```python
from build123d import *

# Parameters (mm, degrees)
SKETCH_1_R          = 1.5
EXTRUDE_1_DEPTH     = 8
SKETCH_2_R          = 1.5
CUT_EXTRUDE_1_DEPTH = 28.367864367
SKETCH_3_R          = 3
CUT_EXTRUDE_2_DEPTH = 3
CUT_EXTRUDE_3_DEPTH = 3


with BuildPart() as part:
    # 草图1 → 凸台-拉伸1 (new body)
    with BuildSketch(Plane(origin=(0, 0, 0), x_dir=(1, 0, 0), z_dir=(0, 1, 0))):
        Polygon((-18, 19), (18, 19), (18, 6), (10, 6), (10, 0), (-10, 0), (-10, 6), (-18, 6), align=None)
        with Locations(Location((7.5, 14.5, 0), (0, 0, 270))):
            Circle(SKETCH_1_R, mode=Mode.SUBTRACT)
        with Locations(Location((7.5, 4.5, 0), (0, 0, 90))):
            Circle(SKETCH_1_R, mode=Mode.SUBTRACT)
        with Locations(Location((-7.5, 4.5, 0), (0, 0, 270))):
            Circle(SKETCH_1_R, mode=Mode.SUBTRACT)
        with Locations(Location((-7.5, 14.5, 0), (0, 0, 90))):
            Circle(SKETCH_1_R, mode=Mode.SUBTRACT)
    extrude(amount=EXTRUDE_1_DEPTH)

    # 草图2 → 切除-拉伸1 (cut, through all)
    with BuildSketch(Plane(origin=(0, 0, -19), x_dir=(-1, 0, 0), z_dir=(0, 0, -1))):
        with Locations((-14, 4)):
            Circle(SKETCH_2_R)
        with Locations((14, 4)):
            Circle(SKETCH_2_R)
    extrude(amount=-CUT_EXTRUDE_1_DEPTH, mode=Mode.SUBTRACT)

    # 草图3 → 切除-拉伸2 (cut)
    with BuildSketch(Plane.XZ):
        with Locations(Location((-7.5, -14.5, 0), (0, 0, 270))):
            Circle(SKETCH_3_R)
        with Locations(Location((7.5, -14.5, 0), (0, 0, 270))):
            Circle(SKETCH_3_R)
    extrude(amount=-CUT_EXTRUDE_2_DEPTH, mode=Mode.SUBTRACT)

    # 草图4 → 切除-拉伸3 (cut)
    with BuildSketch(Plane.XZ):
        with BuildLine():
            ThreePointArc((-10, -2.841687605), (-6.633974596, -1.627718677), (-4.5, -4.5))
            Line((-4.5, -4.5), (-4.5, 0))
            Line((-4.5, 0), (-10, 0))
            Line((-10, 0), (-10, -2.841687605))
        make_face()
        with BuildLine():
            Line((-6, -4.5), (-4.5, -4.5))
            ThreePointArc((-4.5, -4.5), (-6.633974596, -1.627718677), (-10, -2.841687605))
            Line((-10, -2.841687605), (-10, -4.5))
            Line((-10, -4.5), (-9, -4.5))
            ThreePointArc((-9, -4.5), (-7.5, -3), (-6, -4.5))
        make_face()
        with BuildLine():
            ThreePointArc((-10.098076211, -6), (-6.723542865, -7.397777479), (-4.5, -4.5))
            Line((-4.5, -4.5), (-6, -4.5))
            ThreePointArc((-6, -4.5), (-7.5, -6), (-9, -4.5))
            Line((-9, -4.5), (-10, -4.5))
            Line((-10, -4.5), (-10, -6))
            Line((-10, -6), (-10.098076211, -6))
        make_face()
        with BuildLine():
            ThreePointArc((10, -2.841687605), (6.633974596, -1.627718677), (4.5, -4.5))
            Line((4.5, -4.5), (6, -4.5))
            ThreePointArc((6, -4.5), (7.5, -3), (9, -4.5))
            Line((9, -4.5), (10, -4.5))
            Line((10, -4.5), (10, -2.841687605))
        make_face()
        with BuildLine():
            Line((6, -4.5), (4.5, -4.5))
            ThreePointArc((4.5, -4.5), (6.723542865, -7.397777479), (10.098076211, -6))
            Line((10.098076211, -6), (10, -6))
            Line((10, -6), (10, -4.5))
            Line((10, -4.5), (9, -4.5))
            ThreePointArc((9, -4.5), (7.5, -6), (6, -4.5))
        make_face()
        with BuildLine():
            Line((10, 0), (4.5, 0))
            Line((4.5, 0), (4.5, -4.5))
            ThreePointArc((4.5, -4.5), (6.633974596, -1.627718677), (10, -2.841687605))
            Line((10, -2.841687605), (10, 0))
        make_face()
    extrude(amount=-CUT_EXTRUDE_3_DEPTH, mode=Mode.SUBTRACT)


solid = part.part
```
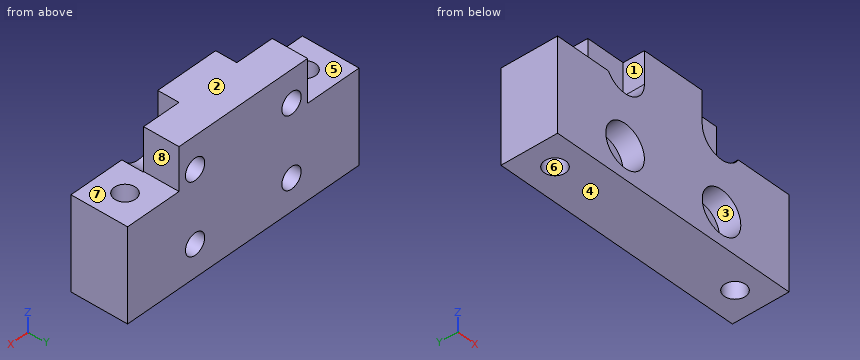
Geometry: final body of the model. Coordinates: model frame, mm. Face numbers are marked on the shaded views. A direction names the side the tool comes from. Round coordinates to 2 decimals unless told otherwise and drop trailing zeros. Write each loop counter-clockwise with the first axis right and the second up, starting at its lowest first coordinate (ties: lowest second). Pieces come first, ordered by that corner, then holes.
Item 1: Mould query, pull axis X, two halves, no side actions, for the marked faces 6, 7 and 8. Classes: +X half, -X half, draft (parallel to the pull), parting line (faces both ways), or undercut.
Item 2: Set-up query: the marked faces 1, 2, 3, 4 and 5. Return all of +Z, -Z, +X, -X, +Y, -Y with unobstructed straight access to the full face (end or side cutting, diameter ignored); none if empty.
Item 3: Material intervals for L1, parallel to Z at x = 7.5, y = 4.5; L2, parallel to X at y = 6.65, z = -4.5; L3, parallel to X at y = 0.8, z = -14.5, sorted ascending.
Item 4: Section query D-D (x = 7.5). Return loops of the section in (y, z).
Item 5: Section query B-B (x = 14). Return loops of the section in (y, z).
Item 6: Section query A-A (y = 4). Return loops of the section in (x, z), plus the area to 3 significant figures.
Item 7: Section query C-C (z = -14.5). Return loops of the section in (x, y), plus the area to 3 significant figures.
Item 8: Pin query (flat end, axial travel): P1, Ø4, axis at x = 3, y = 4, coming from the +Z side; P2, Ø5, axis at x = -7.5, z = -14.5, coming from the -Y side; P3, Ø2.5, axis at x = -7.5, z = -14.5, coming from the +Y side; P4, Ø0.9, axis at y = 2, z = -1.5, coming from the -X side. Return the tip coordinate at first contact, or that it passes through.
Completed:
1. face 6: undercut
1. face 7: draft
1. face 8: +X half
2. face 1: +Z, -X, -Y
2. face 2: +Z, +X, -X, +Y, -Y
2. face 3: -Y
2. face 4: -Z, +X, -X, +Y, -Y
2. face 5: +Z, -X, +Y, -Y
3. L1: z = -19 to -16, -13 to -6, -3 to 0
3. L2: x = -10 to -9, -6 to 6, 9 to 10
3. L3: x = -18 to -10.5, -4.5 to 4.5, 10.5 to 18
4. outline: (0, -19) - (8, -19) - (8, -16) - (3, -16) - (3, -17.5) - (0, -17.5) - close; (0, -11.5) - (3, -11.5) - (3, -13) - (8, -13) - (8, -6) - (3, -6) - (3, -7.5) - (0, -7.5) - close; (3, -3) - (8, -3) - (8, 0) - (3, 0) - close
5. outline: (0, -19) - (2.5, -19) - (2.5, -6) - (0, -6) - close; (5.5, -19) - (8, -19) - (8, -6) - (5.5, -6) - close
6. outline: (-18, -19) - (-15.5, -19) - (-15.5, -6) - (-18, -6) - close; (-12.5, -19) - (12.5, -19) - (12.5, -6) - (10, -6) - (10, 0) - (-10, 0) - (-10, -6) - (-12.5, -6) - close; (15.5, -19) - (18, -19) - (18, -6) - (15.5, -6) - close; hole circle Ø3 at (-7.5, -14.5); hole circle Ø3 at (-7.5, -4.5); hole circle Ø3 at (7.5, -14.5); hole circle Ø3 at (7.5, -4.5)
6. area: 482 mm2
7. outline: (-18, 0) - (-10.5, 0) - (-10.5, 3) - (-9, 3) - (-9, 8) - (-18, 8) - close; (-6, 3) - (-4.5, 3) - (-4.5, 0) - (4.5, 0) - (4.5, 3) - (6, 3) - (6, 8) - (-6, 8) - close; (9, 3) - (10.5, 3) - (10.5, 0) - (18, 0) - (18, 8) - (9, 8) - close; hole circle Ø3 at (-14, 4); hole circle Ø3 at (14, 4)
7. area: 208 mm2
8. P1: stops at z = 0
8. P2: stops at y = 3
8. P3: passes through
8. P4: stops at x = -4.5
